Read the model definition and answer for the solid it produces. Units are mm, in the model's axes. A direction names the side the tool comes from. Coordinates: 2 decimals unless noted, no trailing zeros. Write each loop counter-clockwise with the first axis right and the second up, starting at its lowest first coordinate (ties: lowest second). Pieces come first, ordered by that corner, then holes. Notation, with made-up numbers: (74.5, 45) -> (116.5, 45) arc R22 ccw to (116.5, 80) -> close; hole circle Ø3 at (77.25, -14). An arc over 180 degrees is marked (long way). Answer in a Markdown table with one row per item. Add a question column.
Item 1: For a pull along Z with two mould halves and no side action, classify faces 6 (the face through (-7, -7, 12)), 7 (the face through (26, -27, 51)), 8 (the face through (4, -20, 10)) as +Z half, -Z half, draft (parallel to the pull), parting line (faces both ways), or undercut.
Item 2: Straight lines are drawn through the part: line 1 (X direction, y = -27, z = 53); line 2 (Y direction, x = -17.5, z = 6.5); line 3 (X direction, y = -22, z = 41). For each, find the intervals that lie inside material, in ascending order. Write a range as from..to.
Item 3: Section B-B on y = -27 is taken. Write down the section's boundary in (x, z) (3 decimals), then the cut area to 3 significant figures.
Item 4: Section D-D on x = 25.5 is taken. Write down the section's boundary in (y, z), then the cut area to 3 significant figures.
Item 5: Which of the six approach directions +Z, -Z, +X, -X, +Y, -Y give full straight-line access (tool end or side, diameter ignored) to faces 1 (the face through (-22, -19, 34)), 2 (the face through (15.69, 8.86, 1.97)), 3 (the face through (14, -27, 34)), 4 (the face through (0, -20, 9)), 5 (the face through (20.162, -30.125, 38.675))?
Item 6: Section A-A on z = 23 is taken. Write down the section's boundary in (x, y), then the cut area to 3 significant figures.
Item 7: Section C-C on x = 0 is taken. Write down the section's boundary in (y, z), then the cut area to 3 significant figures.
Item 8: Given pin 1 Ø6 at (x, z) = (-18.5, 18) entering from +Y; pin 2 Ø3 at (y, z) = (-25.5, 41) entering from -X; pin 3 Ø12 at (x, y) = (14, 22.5) entering from +Z, each flat-ended and moving along its own axis, determine where each tip first touches the part or whether it passes through.
Autodesk Fusion 360 part; units mm, degrees
sketch "01 - PRIMARY SUPPORT MECHANISM ( LEFT SIDE ) SKETCH" plane through (0, 0, 0) normal (0, 0, 1) x (1, 0, 0)
  line L0 (0, -35) -> (0, -5.422) construction
  line L1 (13.875, 9.9067) -> (17.5, 7.8138)
  circle A0 centre (17.5, 11.9996) radius 2.14
  line L2 (-13.875, 14.0925) -> (-17.5, 16.1854)
  circle A1 centre (-17.5, 11.9996) radius 2.14
  line L3 (-21.125, 14.0925) -> (-21.125, 9.9067)
  line L4 (4, -5.422) -> (4, -35)
  line L5 (30, 35) -> (30, -35)
  line L6 (-7.6, -5.422) -> (-7.6, 0.1231)
  line L7 (-4, -5.422) -> (-4, -35)
  line L8 (17.5, 7.8138) -> (21.125, 9.9067)
  line L9 (-21.125, 9.9067) -> (-17.5, 7.8138)
  line L10 (7.6, -5.422) -> (7.6, 0.1231)
  line L11 (21.125, 14.0925) -> (17.5, 16.1854)
  line L12 (-30, 35) -> (30, 35)
  line L13 (21.125, 9.9067) -> (21.125, 14.0925)
  line L14 (13.875, 14.0925) -> (13.875, 9.9067)
  line L15 (-17.5, 7.8138) -> (-13.875, 9.9067)
  line L16 (-30, -19) -> (30, -19) construction
  line L17 (30, -35) -> (-30, -35)
  line L18 (17.5, 16.1854) -> (13.875, 14.0925)
  line L19 (-17.5, 11.9996) -> (-17.5, 14.1396) construction
  line L20 (17.5, 11.9996) -> (17.5, 14.1396) construction
  line L21 (-17.5, 11.9996) -> (17.5, 11.9996) construction
  arc A2 (7.6, 0.1231) -> (-7.6, 0.1231) centre (0, 11.9996) ccw
  line L22 (-17.5, 16.1854) -> (-21.125, 14.0925)
  line L23 (-30, -35) -> (-30, 35)
  line L24 (-7.6, -5.422) -> (7.6, -5.422)
  line L25 (-13.875, 9.9067) -> (-13.875, 14.0925)
  point P0 (17.5, 11.9996)
  point P1 (-17.5, 11.9996)
  dimension "d1" = 60
  dimension "d2" = 70
  dimension "d5" = 16
  dimension "d6" = 29.578
  dimension "d7" = 15.2
  dimension "d8" = 5.5451
  dimension "d9" = 14.1
  dimension "d10" = 17.4216
  dimension "d11" = 8
  dimension "d12" = 4
  dimension "d13" = 35
  dimension "d14" = 4.28
  dimension "d15" = 3.625
  dimension "d16" = 4.28
  dimension "d17" = 3.625
  dimension "d19" = 35
  dimension "d20" = 30
extrude "Extrude1" add sketch "01 - PRIMARY SUPPORT MECHANISM ( LEFT SIDE ) SKETCH" along normal blind 12 contours L1 L8 L11 L13 L18 A2 | L1 L2 L3 L4 L5 L6 L7 L8 L9 L10 L11 L12 L13 L15 L17 L18 A2 L22 L23 L24 | L2 L3 L9 L15 A2 L22 | A0 | A1
extrude "Extrude2" add sketch "01 - PRIMARY SUPPORT MECHANISM ( LEFT SIDE ) SKETCH" along normal blind 9 contours L4 L7 L17 L24
sketch "02 - PRIMARY SUPPORT MECHANISM ( LEFT SIDE ) SKETCH" plane through (0, 0, 12) normal (0, 0, 1) x (-1, 0, 0)
  line L0 (-4, 5.422) -> (-4, 35)
  line L1 (-4, 35) -> (-30, 35)
  line L2 (-30, 35) -> (-30, -35)
  line L3 (-30, -35) -> (30, -35)
  line L4 (30, -35) -> (30, 35)
  line L5 (30, 35) -> (4, 35)
  line L6 (4, 35) -> (4, 5.422)
  line L7 (4, 5.422) -> (7.6, 5.422)
  line L8 (7.6, 5.422) -> (7.6, -0.1231)
  arc A0 (-7.6, -0.1231) -> (7.6, -0.1231) centre (0, -11.9996) ccw
  line L9 (-7.6, -0.1231) -> (-7.6, 5.422)
  line L10 (-7.6, 5.422) -> (-4, 5.422)
  line L11 (30, 35) -> (4, 35)
  line L12 (-4, 35) -> (-30, 35)
  line L13 (30, 35) -> (14, 35)
  line L14 (-14, 35) -> (-14, 19)
  line L15 (14, 35) -> (14, 19)
  line L16 (-30, 19) -> (-30, 35)
  line L17 (-30, 35) -> (-14, 35)
  line L18 (30, 19) -> (30, 35)
  line L19 (14, 19) -> (30, 19)
  line L20 (-14, 19) -> (-30, 19)
  dimension "d25" = 16
  dimension "d26" = 16
  dimension "d27" = 16
  dimension "d28" = 16
extrude "Extrude3" add sketch "02 - PRIMARY SUPPORT MECHANISM ( LEFT SIDE ) SKETCH" along normal blind 45 contours L1 L2 L12 L14 L16 L17 L20 | L4 L5 L11 L13 L15 L18 L19
sketch "03 - PRIMARY SUPPORT MECHANISM ( LEFT SIDE ) SKETCH" plane through (0, 0, 57) normal (0, 0, 1) x (-1, 0, 0)
  line L0 (-14, 19) -> (-14, 35)
  line L1 (-14, 35) -> (-30, 35)
  line L2 (-30, 35) -> (-30, 19)
  line L3 (-30, 19) -> (-14, 19)
  line L4 (-14, 35) -> (-30, 35)
  line L5 (-18.375, 29.0929) -> (-22, 31.1858)
  line L6 (-14, 19) -> (-14, 35)
  line L7 (-22, 22.8142) -> (-18.375, 24.9071)
  line L8 (-14, 27) -> (-30, 27) construction
  line L9 (-25.625, 29.0929) -> (-25.625, 24.9071)
  line L10 (-30, 19) -> (-14, 19)
  line L11 (-22, 23.375) -> (-22, 22.8142)
  line L12 (-25.625, 24.9071) -> (-22, 22.8142)
  line L13 (-22, 22.8142) -> (-30, 22.8142)
  line L14 (-18.375, 24.9071) -> (-18.375, 29.0929)
  line L15 (-22, 31.1858) -> (-22, 30.625)
  line L16 (-30, 31.1858) -> (-30, 22.8142)
  line L17 (-30, 35) -> (-30, 19)
  line L18 (-22, 31.1858) -> (-25.625, 29.0929)
  line L19 (-22, 31.1858) -> (-30, 31.1858)
  circle A0 centre (-22, 27) radius 2.14
  line L20 (-22, 19) -> (-22, 35) construction
  point P0 (-22, 27)
  dimension "d34" = 3.625
  dimension "d35" = 4.28
  dimension "d38" = 16
  dimension "d39" = 16
extrude "Extrude4" cut sketch "03 - PRIMARY SUPPORT MECHANISM ( LEFT SIDE ) SKETCH" against normal blind 25 from surface at -6 contours L2 L9 L12 L13 L16 L17 L18 L19 | L5 L7 L9 L12 L14 L18 | A0
extrude "Extrude5" cut sketch "03 - PRIMARY SUPPORT MECHANISM ( LEFT SIDE ) SKETCH" against normal blind 6 contours A0
sketch "04 - PRIMARY SUPPORT MECHANISM ( LEFT SIDE ) SKETCH" plane through (0, 0, 57) normal (0, 0, 1) x (-1, 0, 0)
  line L0 (14, 19) -> (30, 19)
  line L1 (30, 19) -> (30, 35)
  line L2 (30, 35) -> (14, 35)
  line L3 (14, 35) -> (14, 19)
  line L4 (22, 35) -> (22, 19) construction
  line L5 (30, 27) -> (14, 27) construction
  line L6 (22, 31.1858) -> (18.375, 29.0929)
  line L7 (18.375, 24.9071) -> (22, 22.8142)
  line L8 (30, 35) -> (14, 35)
  line L9 (22, 22.8142) -> (30, 22.8142)
  line L10 (30, 19) -> (30, 35)
  line L11 (25.625, 29.0929) -> (22, 31.1858)
  line L12 (30, 31.1858) -> (30, 22.8142)
  line L13 (22, 22.8142) -> (25.625, 24.9071)
  circle A0 centre (22, 27) radius 2.14
  line L14 (18.375, 29.0929) -> (18.375, 24.9071)
  line L15 (22, 31.1858) -> (30, 31.1858)
  line L16 (25.625, 24.9071) -> (25.625, 29.0929)
  line L17 (14, 19) -> (30, 19)
  line L18 (14, 35) -> (14, 19)
  point P0 (22, 27)
  dimension "d47" = 3.625
  dimension "d48" = 4.28
  dimension "d49" = 16
  dimension "d50" = 16
extrude "Extrude6" cut sketch "04 - PRIMARY SUPPORT MECHANISM ( LEFT SIDE ) SKETCH" against normal blind 25 from surface at -6 contours L1 L9 L10 L11 L12 L13 L15 L16 | L6 L7 L11 L13 L14 L16 | A0
extrude "Extrude7" cut sketch "04 - PRIMARY SUPPORT MECHANISM ( LEFT SIDE ) SKETCH" against normal blind 6 contours A0
extrude "Extrude8" cut sketch "01 - PRIMARY SUPPORT MECHANISM ( LEFT SIDE ) SKETCH" along normal blind 12 contours A0 | A1
extrude "Extrude9" cut sketch "01 - PRIMARY SUPPORT MECHANISM ( LEFT SIDE ) SKETCH" along normal blind 4 contours L1 L8 L11 L13 L18 A2 | L2 L3 L9 L15 A2 L22
Results below:
| question | item | result |
|---|---|---|
| 1 | face 6 | +Z half |
| 1 | face 7 | undercut |
| 1 | face 8 | draft |
| 2 | line 1 | x = -30..-24.14, -19.86..-14, 14..19.86, 24.14..30 |
| 2 | line 2 | y = -35..9.86, 14.14..35 |
| 2 | line 3 | x = -30..-14, 14..30 |
| 3 | outline | (-30, 0) -> (30, 0) -> (30, 26) -> (18.375, 26) -> (18.375, 51) -> (19.86, 51) -> (19.86, 57) -> (14, 57) -> (14, 12) -> (4, 12) -> (4, 9) -> (-4, 9) -> (-4, 12) -> (-14, 12) -> (-14, 57) -> (-19.86, 57) -> (-19.86, 51) -> (-18.375, 51) -> (-18.375, 26) -> (-30, 26) -> close; (-30, 51) -> (-24.14, 51) -> (-24.14, 57) -> (-30, 57) -> close; (24.14, 51) -> (30, 51) -> (30, 57) -> (24.14, 57) -> close |
| 3 | area | 1,500 mm2 |
| 4 | outline | (-35, 0) -> (35, 0) -> (35, 12) -> (-19, 12) -> (-19, 57) -> (-35, 57) -> close; hole (-31.19, 26) -> (-22.81, 26) -> (-22.81, 51) -> (-31.19, 51) -> close |
| 4 | area | 1,350 mm2 |
| 5 | face 1 | +Z, +X, -X, +Y |
| 5 | face 2 | -Z |
| 5 | face 3 | +Z, +Y, -Y |
| 5 | face 4 | +Z, -Y |
| 5 | face 5 | +X |
| 6 | outline | (-30, -35) -> (-14, -35) -> (-14, -19) -> (-30, -19) -> close; (14, -35) -> (30, -35) -> (30, -19) -> (14, -19) -> close |
| 6 | area | 512 mm2 |
| 7 | outline | (-35, 0) -> (-5.42, 0) -> (-5.42, 9) -> (-35, 9) -> close; (26.1, 0) -> (35, 0) -> (35, 12) -> (26.1, 12) -> close |
| 7 | area | 373 mm2 |
| 8 | pin 1 | stops at y = -19 |
| 8 | pin 2 | stops at x = -19.95 |
| 8 | pin 3 | stops at z = 12 |
